Check sheet for the modelled part. Datum: model origin and axes. Units: mm. A direction names the side the tool comes from. Give positions to 0.01 mm unless a question says otherwise; leave off trailing zeros. Loops run counter-clockwise (first coordinate to the right, second up) from the corner with the lowest first, then second, coordinate; pieces in that order, holes last. Notation, with made-up numbers: M -4.75,81.5 L 46.25,81.5 A11 ccw 46.25,87.5 Z; hole C 29.5,-13.5 d4. An arc over 180 degrees is marked long. One line per question, with ' | ' between items. Start each with the question number.
from build123d import *

# Parameters (mm, degrees)
SM_START               = -138.5
SM_BASE_FLANGE_1_DEPTH = 277
SKETCH_6_R             = 59
SKETCH_6_R_2           = 3
SKETCH_6_R_3           = 3.5
CUT_EXTRUDE_1_DEPTH    = 156.647839689


# Read off the part's stored shape, not the designer's step: 基体-法兰1
with BuildPart() as part:
    # 基体-法兰1 outline → 基体-法兰1 (new body)
    with BuildSketch(Plane(origin=(0, 0, 0), x_dir=(0, 0, -1), z_dir=(1, 0, 0)).offset(SM_START)):
        with BuildLine():
            Line((68.5, -1.5), (68.5, -12))
            Line((68.5, -12), (70, -12))
            Line((70, -12), (70, -1.5))
            ThreePointArc((70, -1.5), (69.560660172, -0.439339828), (68.5, 0))
            Line((68.5, 0), (-68.5, 0))
            ThreePointArc((-68.5, 0), (-69.560660172, -0.439339828), (-70, -1.5))
            Line((-70, -1.5), (-70, -12))
            Line((-70, -12), (-68.5, -12))
            Line((-68.5, -12), (-68.5, -1.5))
            Line((-68.5, -1.5), (68.5, -1.5))
        make_face()
    extrude(amount=SM_BASE_FLANGE_1_DEPTH)

    # 草图6 → 切除-拉伸1 (cut, through all)
    with BuildSketch(Plane(origin=(0, 0, 0), x_dir=(1, 0, 0), z_dir=(0, 1, 0))):
        with Locations(Location((-66, 0, 0), (0, 0, 270))):
            Circle(SKETCH_6_R)
        with Locations(Location((-118.5, 52.5, 0), (0, 0, 270))):
            Circle(SKETCH_6_R_2)
        with Locations(Location((-13.5, 52.5, 0), (0, 0, 270))):
            Circle(SKETCH_6_R_2)
        with Locations(Location((-13.5, -52.5, 0), (0, 0, 270))):
            Circle(SKETCH_6_R_2)
        with Locations(Location((-118.5, -52.5, 0), (0, 0, 270))):
            Circle(SKETCH_6_R_2)
        with Locations(Location((125.5, 52.5, 0), (0, 0, 270))):
            Circle(SKETCH_6_R_3)
        with Locations(Location((125.5, -52.5, 0), (0, 0, 270))):
            Circle(SKETCH_6_R_3)
    extrude(amount=-CUT_EXTRUDE_1_DEPTH, mode=Mode.SUBTRACT)


solid = part.part
Q1. Depth check by flat-ended pin: P1, Ø4, axis at x = 125.5, z = -52.5, coming from the +Y side (3 decimals); P2, Ø9, axis at x = 125.5, z = 52.5, coming from the -Y side. Enter the tip coordinate at first touch or a pass-through.
Q2. Material ranges on probe 1 along X at (y, z) = (-0.8, -52.5); probe 2 along Z at (x, y) = (82, -2.5); probe 3 along Y at (x, z) = (63.5, 38), recorded low to high. Write a range as from..to.
Q3. Cross-section at D-D (x = 125.5). Record the cut outline in (y, z), and give its area (3 significant figures).
Q4. Draft check along Z on faces 3 (the cylindrical face through (123.4, -0.7, -55.3)), 4 (the flat face through (29, 0, -1)), 5 (the flat face through (-2, -7, 70)), 6 (the cylindrical face through (-13.4, -0.7, 49.5)). Enter one of: released by +Z, released by -Z, zero draft, split by the parting line, or undercut.
Q5. Cross-section at A-A (x = -66). Record the cut outline in (y, z).
Q6. Cross-section at B-B (z = 0). Record the cut outline in (x, y), and give its area (4 significant figures).
Q7. Access from +Z, -Z, +X, -X, +Y, -Y to the whole of each face (thin tool, end or side, straight path). Record for faces 1 (the flat face through (29, -1.5, 1)), 2 (the cylindrical face through (123.4, -0.7, 49.7)).
Q8. Cross-section at C-C (y = -6.5). Record the cut outline in (x, z).
Solved:
1) P1: passes through | P2: stops at y = -1.5
2) probe 1: x = -138.5..-121.5, -115.5..-92.92, -39.08..-16.5, -10.5..122, 129..138.5 | probe 2: z = -70..-68.5, 68.5..70 | probe 3: y = -1.5..0
3) outline: M -12,-70 L -1.5,-70 A1.5 ccw 0,-68.5 L 0,-56 L -1.5,-56 L -1.5,-68.5 L -12,-68.5 Z; M -12,68.5 L -1.5,68.5 L -1.5,56 L 0,56 L 0,68.5 A1.5 ccw -1.5,70 L -12,70 Z; M -1.5,-49 L 0,-49 L 0,49 L -1.5,49 Z | area: 220 mm²
4) face 3: undercut | face 4: zero draft | face 5: released by +Z | face 6: undercut
5) outline: M -12,-70 L -1.5,-70 A1.5 ccw 0,-68.5 L 0,-59 L -1.5,-59 L -1.5,-68.5 L -12,-68.5 Z; M -12,68.5 L -1.5,68.5 L -1.5,59 L 0,59 L 0,68.5 A1.5 ccw -1.5,70 L -12,70 Z
6) outline: M -138.5,-1.5 L -125,-1.5 L -125,0 L -138.5,0 Z; M -7,-1.5 L 138.5,-1.5 L 138.5,0 L -7,0 Z | area: 238.5 mm²
7) face 1: +X, -X, -Y | face 2: +Y, -Y
8) outline: M -138.5,-70 L 138.5,-70 L 138.5,-68.5 L -138.5,-68.5 Z; M -138.5,68.5 L 138.5,68.5 L 138.5,70 L -138.5,70 Z
